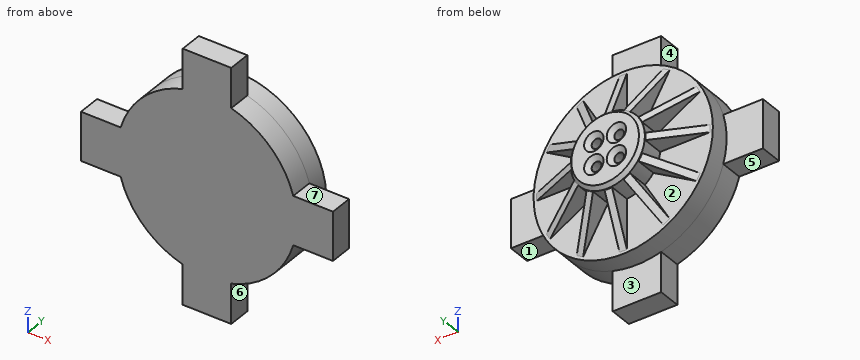
from build123d import *

# Parameters (mm, degrees)
SALIENTE_EXTRUIR1_DEPTH         = 7
CROQUIS2_R                      = 27.75
SALIENTE_EXTRUIR2_DEPTH         = 6
CROQUIS3_R                      = 11.5
SALIENTE_EXTRUIR3_DEPTH         = 6.7
NERVIO5_START                   = -19.605376538
NERVIO5_OUTLINE_W               = 2.3
NERVIO5_OUTLINE_H               = 7.43309969
NERVIO5_DEPTH                   = 16.688717133
MATRIZC1_COUNT                  = 12
CROQUIS5_R                      = 8.65
SALIENTE_EXTRUIR4_DEPTH         = 1.2
CHAFL_N1_SIZE                   = 2.9
CHAFL_N1_SIZE_2                 = 3.2
CORTAR_EXTRUIR1_DEPTH           = 12.6
CROQUIS7_R                      = 3
CORTAR_EXTRUIR2_DEPTH           = 1.2
CORTAR_EXTRUIR2_DRAFT           = -51
CORTAR_EXTRUIR2_PROFILE_2_DEPTH = 1.2
CORTAR_EXTRUIR2_PROFILE_2_DRAFT = -51
CORTAR_EXTRUIR2_PROFILE_3_DEPTH = 1.2
CORTAR_EXTRUIR2_PROFILE_3_DRAFT = -51
CORTAR_EXTRUIR2_PROFILE_4_DEPTH = 1.2
CORTAR_EXTRUIR2_PROFILE_4_DRAFT = -51


# Read off the part's stored shape, not the designer's step: Nervio5
with BuildPart() as part:
    # Croquis1 → Saliente-Extruir1 (new body)
    with BuildSketch(Plane(origin=(0, 0, 0), x_dir=(1, 0, 0), z_dir=(0, 1, 0))):
        with BuildLine():
            Line((-7.5, -39), (7.5, -39))
            Line((7.5, -39), (7.5, -26.717269696))
            ThreePointArc((7.5, -26.717269696), (19.622213178, -19.622213178), (26.717269696, -7.5))
            Line((26.717269696, -7.5), (39, -7.5))
            Line((39, -7.5), (39, 7.5))
            Line((39, 7.5), (26.717269696, 7.5))
            ThreePointArc((26.717269696, 7.5), (19.622213178, 19.622213178), (7.5, 26.717269696))
            Line((7.5, 26.717269696), (7.5, 39))
            Line((7.5, 39), (-7.5, 39))
            Line((-7.5, 39), (-7.5, 26.717269696))
            ThreePointArc((-7.5, 26.717269696), (-19.622213178, 19.622213178), (-26.717269696, 7.5))
            Line((-26.717269696, 7.5), (-39, 7.5))
            Line((-39, 7.5), (-39, -7.5))
            Line((-39, -7.5), (-26.717269696, -7.5))
            ThreePointArc((-26.717269696, -7.5), (-19.622213178, -19.622213178), (-7.5, -26.717269696))
            Line((-7.5, -26.717269696), (-7.5, -39))
        make_face()
    extrude(amount=SALIENTE_EXTRUIR1_DEPTH)

    # Croquis2 → Saliente-Extruir2 (add)
    with BuildSketch(Plane(origin=(0, 7, 0), x_dir=(1, 0, 0), z_dir=(0, 1, 0))):
        with Locations(Location((0, 0, 0), (0, 0, 105.680350135))):
            Circle(CROQUIS2_R)
    extrude(amount=SALIENTE_EXTRUIR2_DEPTH)

    # Croquis3 → Saliente-Extruir3 (add)
    with BuildSketch(Plane(origin=(0, 13, 0), x_dir=(1, 0, 0), z_dir=(0, 1, 0))):
        with Locations(Location((0, 0, 0), (0, 0, 270))):
            Circle(CROQUIS3_R)
    extrude(amount=SALIENTE_EXTRUIR3_DEPTH)

    # Nervio5 outline → Nervio5 (add)
    with BuildSketch(Plane(origin=(0, 0, 0), x_dir=(1, 0, 0), z_dir=(0, 0.39036530164811784, 0.9206600519568415)).offset(NERVIO5_START)):
        with Locations((0, 18.716549845)):
            Rectangle(NERVIO5_OUTLINE_W, NERVIO5_OUTLINE_H)
    nervio5 = extrude(amount=NERVIO5_DEPTH)

    # MatrizC1: Nervio5 ×12 about axis
    matrizc1_axis = Axis((0, 0, 0), (0, 1, 0))
    for i in range(1, MATRIZC1_COUNT):
        add(nervio5.rotate(matrizc1_axis, i * 360 / MATRIZC1_COUNT))

    # Croquis5 → Saliente-Extruir4 (add)
    with BuildSketch(Plane(origin=(0, 19.7, 0), x_dir=(1, 0, 0), z_dir=(0, 1, 0))):
        with Locations(Location((0, 0, 0), (0, 0, 270))):
            Circle(CROQUIS5_R)
    extrude(amount=SALIENTE_EXTRUIR4_DEPTH)

    # Chaflán1
    # the kernel refuses this chamfer: 3.2, 2.9 mm, written as the material it adds along each edge
    with BuildSketch(Plane(origin=(0, 19.7, 0), x_dir=(0, 0, 1), z_dir=(-1, 0, 0))) as chafl_n1_piece_1_section:
        Polygon((8.65 + CHAFL_N1_SIZE, 0), (8.65, CHAFL_N1_SIZE_2), (8.65, 0), align=None)
    chafl_n1_piece_1 = revolve(axis=Axis((0, 19.7, 0), (0, 1, 0)), mode=Mode.PRIVATE)
    chafl_n1_piece_1 = chafl_n1_piece_1 & Plane(origin=(0, 20.288796189, 0), x_dir=(0, 0, 1), z_dir=(0, -1, 0)) * Cylinder(11.5, 47, mode=Mode.PRIVATE)
    chafl_n1_piece_1 = split(chafl_n1_piece_1, bisect_by=Plane(origin=(0, 20.9, -10.938447221), z_dir=(0, -1, 0)), keep=Keep.TOP, mode=Mode.PRIVATE)
    add(chafl_n1_piece_1)

    # Croquis6 → Cortar-Extruir1 (cut)
    with BuildSketch(Plane(origin=(0, 20.9, 0), x_dir=(1, 0, 0), z_dir=(0, 1, 0))):
        with BuildLine():
            ThreePointArc((-2, 3.5), (-4.560660172, 4.560660172), (-3.5, 2))
            Line((-3.5, 2), (-3.5, 3.5))
            Line((-3.5, 3.5), (-2, 3.5))
        make_face()
        with BuildLine():
            Line((-3.5, 3.5), (-3.5, 2))
            ThreePointArc((-3.5, 2), (-2.439339828, 2.439339828), (-2, 3.5))
            Line((-2, 3.5), (-3.5, 3.5))
        make_face()
        with BuildLine():
            ThreePointArc((2, 3.5), (2.439339828, 2.439339828), (3.5, 2))
            Line((3.5, 2), (3.5, 3.5))
            Line((3.5, 3.5), (2, 3.5))
        make_face()
        with BuildLine():
            Line((3.5, 3.5), (3.5, 2))
            ThreePointArc((3.5, 2), (4.560660172, 2.439339828), (5, 3.5))
            ThreePointArc((5, 3.5), (3.5, 5), (2, 3.5))
            Line((2, 3.5), (3.5, 3.5))
        make_face()
        with BuildLine():
            ThreePointArc((3.5, -2), (2.439339828, -2.439339828), (2, -3.5))
            Line((2, -3.5), (3.5, -3.5))
            Line((3.5, -3.5), (3.5, -2))
        make_face()
        with BuildLine():
            Line((3.5, -3.5), (2, -3.5))
            ThreePointArc((2, -3.5), (3.5, -5), (5, -3.5))
            ThreePointArc((5, -3.5), (4.560660172, -2.439339828), (3.5, -2))
            Line((3.5, -2), (3.5, -3.5))
        make_face()
        with BuildLine():
            Line((-3.5, -2), (-3.5, -3.5))
            Line((-3.5, -3.5), (-2, -3.5))
            ThreePointArc((-2, -3.5), (-2.439339828, -2.439339828), (-3.5, -2))
        make_face()
        with BuildLine():
            Line((-2, -3.5), (-3.5, -3.5))
            Line((-3.5, -3.5), (-3.5, -2))
            ThreePointArc((-3.5, -2), (-4.560660172, -4.560660172), (-2, -3.5))
        make_face()
    extrude(amount=-CORTAR_EXTRUIR1_DEPTH, mode=Mode.SUBTRACT)


with BuildPart() as cortar_extruir2_tool:
    # Croquis7 → Cortar-Extruir2 (with draft: the straight prism first)
    with BuildSketch(Plane(origin=(0, 20.9, 0), x_dir=(1, 0, 0), z_dir=(0, 1, 0))):
        with Locations((-3.5, 3.5)):
            Circle(CROQUIS7_R)
    extrude(amount=-CORTAR_EXTRUIR2_DEPTH)
    # Cortar-Extruir2: the draft: its side faces are tilted about the plane it starts from
    cortar_extruir2_sides = [cortar_extruir2_tool.faces().sort_by_distance(p)[0] for p in [
        (-6.5, 20.3, -3.5),
    ]]
    draft(cortar_extruir2_sides, Plane(origin=(0, 20.9, 0), x_dir=(1, 0, 0), z_dir=(0, 1, 0)), CORTAR_EXTRUIR2_DRAFT)


with BuildPart() as part_1:
    add(part.part)

    # Cortar-Extruir2: cut by cortar_extruir2_tool
    add(cortar_extruir2_tool.part, mode=Mode.SUBTRACT)


with BuildPart() as cortar_extruir2_profile_2_tool:
    # Croquis7 → Cortar-Extruir2 profile 2 (with draft: the straight prism first)
    with BuildSketch(Plane(origin=(0, 20.9, 0), x_dir=(1, 0, 0), z_dir=(0, 1, 0))):
        with Locations((3.5, 3.5)):
            Circle(CROQUIS7_R)
    extrude(amount=-CORTAR_EXTRUIR2_PROFILE_2_DEPTH)
    # Cortar-Extruir2 profile 2: the draft: its side faces are tilted about the plane it starts from
    cortar_extruir2_profile_2_sides = [cortar_extruir2_profile_2_tool.faces().sort_by_distance(p)[0] for p in [
        (0.5, 20.3, -3.5),
    ]]
    draft(cortar_extruir2_profile_2_sides, Plane(origin=(0, 20.9, 0), x_dir=(1, 0, 0), z_dir=(0, 1, 0)), CORTAR_EXTRUIR2_PROFILE_2_DRAFT)


with BuildPart() as part_2:
    add(part_1.part)

    # Cortar-Extruir2 profile 2: cut by cortar_extruir2_profile_2_tool
    add(cortar_extruir2_profile_2_tool.part, mode=Mode.SUBTRACT)


with BuildPart() as cortar_extruir2_profile_3_tool:
    # Croquis7 → Cortar-Extruir2 profile 3 (with draft: the straight prism first)
    with BuildSketch(Plane(origin=(0, 20.9, 0), x_dir=(1, 0, 0), z_dir=(0, 1, 0))):
        with Locations((3.5, -3.5)):
            Circle(CROQUIS7_R)
    extrude(amount=-CORTAR_EXTRUIR2_PROFILE_3_DEPTH)
    # Cortar-Extruir2 profile 3: the draft: its side faces are tilted about the plane it starts from
    cortar_extruir2_profile_3_sides = [cortar_extruir2_profile_3_tool.faces().sort_by_distance(p)[0] for p in [
        (0.5, 20.3, 3.5),
    ]]
    draft(cortar_extruir2_profile_3_sides, Plane(origin=(0, 20.9, 0), x_dir=(1, 0, 0), z_dir=(0, 1, 0)), CORTAR_EXTRUIR2_PROFILE_3_DRAFT)


with BuildPart() as part_3:
    add(part_2.part)

    # Cortar-Extruir2 profile 3: cut by cortar_extruir2_profile_3_tool
    add(cortar_extruir2_profile_3_tool.part, mode=Mode.SUBTRACT)


with BuildPart() as cortar_extruir2_profile_4_tool:
    # Croquis7 → Cortar-Extruir2 profile 4 (with draft: the straight prism first)
    with BuildSketch(Plane(origin=(0, 20.9, 0), x_dir=(1, 0, 0), z_dir=(0, 1, 0))):
        with Locations((-3.5, -3.5)):
            Circle(CROQUIS7_R)
    extrude(amount=-CORTAR_EXTRUIR2_PROFILE_4_DEPTH)
    # Cortar-Extruir2 profile 4: the draft: its side faces are tilted about the plane it starts from
    cortar_extruir2_profile_4_sides = [cortar_extruir2_profile_4_tool.faces().sort_by_distance(p)[0] for p in [
        (-6.5, 20.3, 3.5),
    ]]
    draft(cortar_extruir2_profile_4_sides, Plane(origin=(0, 20.9, 0), x_dir=(1, 0, 0), z_dir=(0, 1, 0)), CORTAR_EXTRUIR2_PROFILE_4_DRAFT)


with BuildPart() as part_4:
    add(part_3.part)

    # Cortar-Extruir2 profile 4: cut by cortar_extruir2_profile_4_tool
    add(cortar_extruir2_profile_4_tool.part, mode=Mode.SUBTRACT)


solid = part_4.part
Check sheet for the modelled part. Datum: model origin and axes. Units: mm. Face numbers are marked on the shaded views. A direction names the side the tool comes from. Give positions to 0.01 mm unless a question says otherwise; leave off trailing zeros. Order: outer loops, then holes, each group sorted by start corner. A loop starts at its lowest first (then second) coordinate and runs counter-clockwise, first axis right, second up. Notation, with made-up numbers: M 43.5,41.5 L 74.5,41.5 A23 ccw 74.5,73.5 Z; hole C 25.25,80 d5. An arc over 180 degrees is marked long. Answer as CSV lines item,"result". Start each with the question number.
Item 1: Cross-section at D-D on z = -32. Enter the section's corners in (x, y).
Item 2: Gauge pin test, flat ends, axial feed: P1, Ø10, axis at x = -35.5, z = -2.5, coming from the +Y side; P2, Ø8, axis at y = 2.5, z = 28, coming from the -X side; P3, Ø12, axis at x = 13, y = 15, coming from the +Z side. Record the tip position at first contact, or that the pin passes through.
Item 3: Cross-section at A-A on x = -20. Enter the section's corners in (y, z), plus the area to 3 significant figures.
Item 4: Cross-section at C-C on y = 16. State how many separate pieces and enclosed holes the cut face has, plus the area to 3 significant figures.
Item 5: Tool access check on the marked faces 4, 5, 6 and 7. Record the directions out of +Z, -Z, +X, -X, +Y, -Y that give a thin tool (end or side, any length) a straight path to the whole face; none if there is none.
Item 6: Mould release check, pull along Z, two halves, no side actions. Record for the marked faces 1, 2 and 3: +Z half, -Z half, draft (parallel to the pull), parting line (faces both ways), or undercut.
Item 7: Cross-section at B-B on z = -21.5. Enter the section's corners in (x, y).
Item 8: Thickness scan on line 1 (Z direction, x = -3.5, y = 17.25); line 2 (X direction, y = 12, z = 3.5). Record the ranges inside material, lowest first. Write a range as [from, to].
Established:
1,outline,"M -7.5,0 L 7.5,0 L 7.5,7 L -7.5,7 Z"
2,P1,"stops at y = 7"
2,P2,"stops at x = -13.93"
2,P3,"stops at z = 26.76"
3,outline,"M 0,-19.24 L 13,-19.24 L 13,-12.87 L 14.29,-12.87 L 14.86,-10.22 L 13,-10.22 L 13,-1.15 L 15.89,-1.15 L 15.89,1.15 L 13,1.15 L 13,10.22 L 14.86,10.22 L 14.29,12.87 L 13,12.87 L 13,19.24 L 0,19.24 Z"
3,area,"515 mm^2"
4,separate pieces,"1"
4,enclosed holes,"4"
4,area,"615 mm^2"
5,face 4,"+Z, -X, +Y, -Y"
5,face 5,"-Z, -X, +Y, -Y"
5,face 6,"-Z, +X, +Y, -Y"
5,face 7,"+Z, +X, +Y, -Y"
6,face 1,"-Z half"
6,face 2,"undercut"
6,face 3,"draft"
7,outline,"M -17.54,0 L 17.54,0 L 17.54,13 L 13.74,13 L 13.74,13.56 L 11.09,14.12 L 11.09,13 L 1.15,13 L 1.15,15.25 L -1.15,15.25 L -1.15,13 L -11.09,13 L -11.09,14.12 L -13.74,13.56 L -13.74,13 L -17.54,13 Z"
8,line 1,"z = [-10.95, -5], [-2, 2], [5, 10.95]"
8,line 2,"x = [-27.53, -5], [-2, 2], [5, 27.53]"
